The model under review builds one solid part; all positions refer to its coordinate system, in mm. Coordinates: 2 decimals unless noted, no trailing zeros. Loops run counter-clockwise (first coordinate to the right, second up) from the corner with the lowest first, then second, coordinate; pieces in that order, holes last. Notation, with made-up numbers: (8.25, -13) - (46.25, -13) arc R20 ccw to (46.25, -4) - close; hole circle Ø5 at (-25, -22.75). An arc over 180 degrees is marked (long way). Use a Markdown table: item, result. Add a question column.
1) To check wall thickness, follow L1, parallel to X at y = -25.9, z = 25; L2, parallel to Z at x = 60, y = -25.8; L3, parallel to X at y = -26.25, z = 10. State the ranges of each line that lie inside material, in increasing order. Write a range as [from, to].
2) Add section C-C, the plane y = -25.85. Give the boundary of the cut face in (x, z).
3) Add section D-D, the plane z = 4. Give the boundary of the cut face in (x, y).
4) Clearance check with a flat-ended pin moving along its axis: pin 1 (5 mm diameter, centred on x = 60, z = 25, fed in from +Y). State where the tip first meets the part, or that it passes through.
5) The part is to be moulded in two halves that separate along X. For faces 1 (the flat face through (60, -26, -31)), 2 (the flat face through (-1, -25.3, 0)), 3 (the cylindrical face through (-61.43, -26.21, -25.45)), say which applies: pulls with the +X half, pulls with the -X half, needs draft (parallel to the pull), parting line crosses it, or undercut.
6) Add section B-B, the plane x = 60. Give the boundary of the cut face in (y, z), and give its area (3 significant figures).
7) Add section A-A, the plane z = 25. Give the boundary of the cut face in (x, y).
```python
from build123d import *

# Parameters (mm, degrees)
SKETCH1_W                = 128
SKETCH1_H                = 70
BOSS_EXTRUDE1_DEPTH      = 1.6
CHAMFER1_SIZE            = 8
F_3_0_3_DIAMETER_HOLE1_D = 3
SKETCH4_W                = 95
SKETCH4_H                = 62
BOSS_EXTRUDE2_DEPTH      = 0.1
SKETCH5_W                = 6.5
SKETCH5_H                = 25
CUT_EXTRUDE1_DEPTH       = 2.7


with BuildPart() as part:
    # Sketch1 → Boss-Extrude1 (new body)
    with BuildSketch(Plane(origin=(0, -27, 0), x_dir=(1, 0, 0), z_dir=(0, 1, 0))):
        Rectangle(SKETCH1_W, SKETCH1_H)
    extrude(amount=BOSS_EXTRUDE1_DEPTH)

    # Chamfer1
    chamfer1_edges = [part.edges().sort_by_distance(p)[0] for p in [
        (64, -26.2, 35),
        (-64, -26.2, 35),
        (-64, -26.2, -35),
        (64, -26.2, -35),
    ]]
    chamfer(chamfer1_edges, length=CHAMFER1_SIZE)

    # Ø3.0 (3) Diameter Hole1 (through all)
    with Locations(Plane(origin=(0, -25.4, 0), x_dir=(1, 0, 0), z_dir=(0, 1, 0))):
        with Locations((-60, -25), (-60, 25), (60, 25), (60, -25)):
            Hole(F_3_0_3_DIAMETER_HOLE1_D / 2)

    # Sketch4 → Boss-Extrude2 (add)
    with BuildSketch(Plane(origin=(0, -25.4, 0), x_dir=(1, 0, 0), z_dir=(0, 1, 0))):
        Rectangle(SKETCH4_W, SKETCH4_H)
    extrude(amount=BOSS_EXTRUDE2_DEPTH)

    # Sketch5 → Cut-Extrude1 (cut, through all)
    with BuildSketch(Plane.XZ.offset(27)):
        with Locations((-19.25, 0)):
            Rectangle(SKETCH5_W, SKETCH5_H)
    extrude(amount=-CUT_EXTRUDE1_DEPTH, mode=Mode.SUBTRACT)


solid = part.part
```
From the geometry:
| question | item | result |
|---|---|---|
| 1 | L1 | x = [-64, -61.5], [-58.5, 58.5], [61.5, 64] |
| 1 | L2 | z = [-31, -26.5], [-23.5, 23.5], [26.5, 31] |
| 1 | L3 | x = [-64, -22.5], [-16, 64] |
| 2 | outline | (-64, -27) - (-56, -35) - (56, -35) - (64, -27) - (64, 27) - (56, 35) - (-56, 35) - (-64, 27) - close; hole circle Ø3 at (-60, -25); hole circle Ø3 at (-60, 25); hole (-22.5, -12.5) - (-16, -12.5) - (-16, 12.5) - (-22.5, 12.5) - close; hole circle Ø3 at (60, -25); hole circle Ø3 at (60, 25) |
| 3 | outline | (-64, -27) - (-22.5, -27) - (-22.5, -25.3) - (-47.5, -25.3) - (-47.5, -25.4) - (-64, -25.4) - close; (-16, -27) - (64, -27) - (64, -25.4) - (47.5, -25.4) - (47.5, -25.3) - (-16, -25.3) - close |
| 4 | pin 1 | stops at y = -25.4 |
| 5 | face 1 | pulls with the +X half |
| 5 | face 2 | needs draft |
| 5 | face 3 | undercut |
| 6 | outline | (-27, -31) - (-25.4, -31) - (-25.4, -26.5) - (-27, -26.5) - close; (-27, -23.5) - (-25.4, -23.5) - (-25.4, 23.5) - (-27, 23.5) - close; (-27, 26.5) - (-25.4, 26.5) - (-25.4, 31) - (-27, 31) - close |
| 6 | area | 89.6 mm^2 |
| 7 | outline | (-64, -27) - (-61.5, -27) - (-61.5, -25.4) - (-64, -25.4) - close; (-58.5, -27) - (58.5, -27) - (58.5, -25.4) - (47.5, -25.4) - (47.5, -25.3) - (-47.5, -25.3) - (-47.5, -25.4) - (-58.5, -25.4) - close; (61.5, -27) - (64, -27) - (64, -25.4) - (61.5, -25.4) - close |
